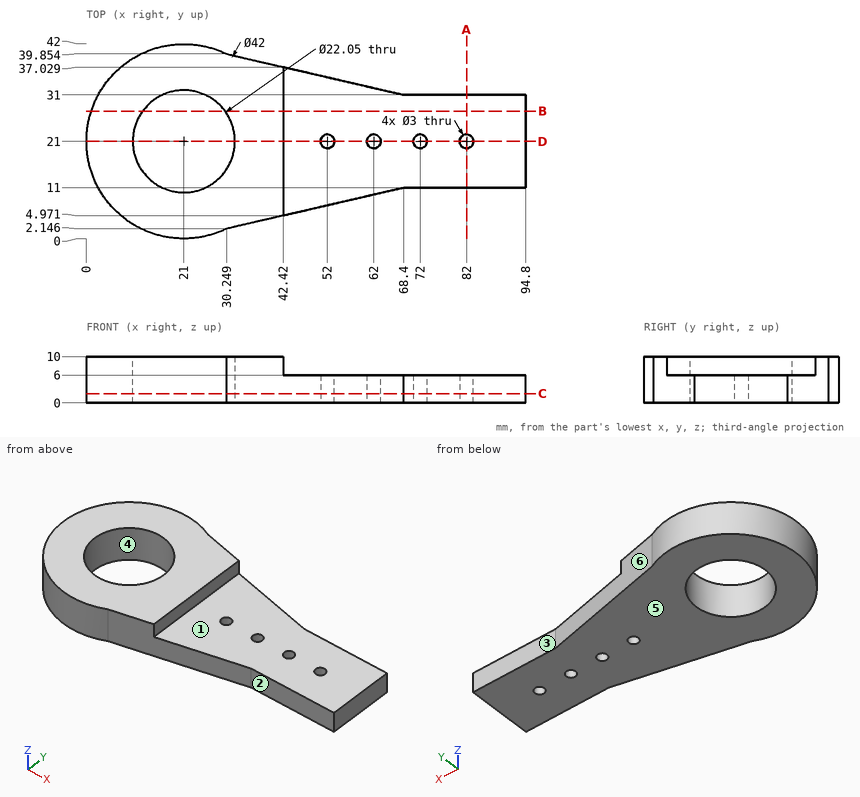
Check sheet for the drawn part. Datum: minimum x, y, z corner. Units: mm. A direction names the side the tool comes from. Coordinates: 2 decimals unless noted, no trailing zeros. Write each loop counter-clockwise with the first axis right and the second up, starting at its lowest first coordinate (ties: lowest second). Pieces come first, ordered by that corner, then holes. Notation, with made-up numbers: (23, -20) - (77, -20) arc R17 cw to (77, -10) - close; hole circle Ø1 at (82.25, 56). An arc over 180 degrees is marked (long way). Answer as a JSON object with one key per item and string values.
(1) Cross-section at C-C on z = 2. Give the number of separate pieces and of enclosed holes in the cut face, plus the area to 3 significant figures.
Report:
{"separate pieces": "1", "enclosed holes": "5", "area": "2,290 mm^2"}
(2) Cross-section at B-B on y = 27.5. Record the cut outline in (x, z) (1 decimal).
Report:
{"outline": "(1, 0) - (12.1, 0) - (12.1, 10) - (1, 10) - close; (29.9, 0) - (94.8, 0) - (94.8, 6) - (42.4, 6) - (42.4, 10) - (29.9, 10) - close"}
(3) Tool access check on the marked faces 1, 2 and 3. Record the directions out of +Z, -Z, +X, -X, +Y, -Y that give a thin tool (end or side, any length) a straight path to the whole face; none if there is none.
Report:
{"face 1": "+Z, +X, +Y, -Y", "face 2": "+Z, -Z, +X, -Y", "face 3": "+Z, -Z, +X, +Y"}
(4) Thickness scan on line 1 along X through (y, z) = (21, 3.9) (1 decimal); line 2 along Y through (x, z) = (72, 2.4); line 3 along X through (y, z) = (21, 8) (1 decimal). Record the ranges inside material, lowest first.
Report:
{"line 1": "0 to 10, 32 to 50.5, 53.5 to 60.5, 63.5 to 70.5, 73.5 to 80.5, 83.5 to 94.8", "line 2": "11 to 19.5, 22.5 to 31", "line 3": "0 to 10, 32 to 42.4"}
(5) Cross-section at D-D on y = 21. Record the cut outline in (x, z) (1 decimal), plus the area to 3 significant figures.
Report:
{"outline": "(0, 0) - (10, 0) - (10, 10) - (0, 10) - close; (32, 0) - (50.5, 0) - (50.5, 6) - (42.4, 6) - (42.4, 10) - (32, 10) - close; (53.5, 0) - (60.5, 0) - (60.5, 6) - (53.5, 6) - close; (63.5, 0) - (70.5, 0) - (70.5, 6) - (63.5, 6) - close; (73.5, 0) - (80.5, 0) - (80.5, 6) - (73.5, 6) - close; (83.5, 0) - (94.8, 0) - (94.8, 6) - (83.5, 6) - close", "area": "446 mm^2"}
(6) Cross-section at A-A on x = 82. Record the cut outline in (y, z), plus the area to 3 significant figures.
Report:
{"outline": "(11, 0) - (19.5, 0) - (19.5, 6) - (11, 6) - close; (22.5, 0) - (31, 0) - (31, 6) - (22.5, 6) - close", "area": "102 mm^2"}
(7) Gauge pin test, flat ends, axial feed: pin 1 Ø2.5 at (x, y) = (52, 21) entering from -Z; pin 2 Ø1 at (y, z) = (10, 7) entering from +X; pin 3 Ø5 at (x, y) = (82, 21) entering from +Z; pin 4 Ø5 at (x, z) = (82.5, 3.5) entering from -Y. Record the tip position at first contact, or that the pin passes through.
Report:
{"pin 1": "through", "pin 2": "x = 42.42", "pin 3": "z = 6", "pin 4": "y = 11"}
(8) Mould release check, pull along X, two halves, no side actions. Record for the marked faces 4, 5 and 6: pulls with the +X half, pulls with the -X half, needs draft (parallel to the pull), parting line crosses it, or undercut.
Report:
{"face 4": "undercut", "face 5": "needs draft", "face 6": "pulls with the +X half"}
